Work out the finished part from the listing and answer in its coordinate system (mm). A direction names the side the tool comes from. Round coordinates to 2 decimals unless told otherwise and drop trailing zeros. Order: outer loops, then holes, each group sorted by start corner. A loop starts at its lowest first (then second) coordinate and runs counter-clockwise, first axis right, second up. Notation, with made-up numbers: (32.25, -3.75) - (70.25, -3.75) arc R24 ccw to (70.25, 26.25) - close; hole circle Ø10 at (66.25, 69). An arc over 180 degrees is marked (long way). Answer in a Markdown table with one row per item.
Autodesk Inventor part; units mm, degrees
ref_plane "YZ Plane" through (0, 0, 0) normal (1, 0, 0) x (0, 1, 0)
ref_plane "XZ Plane" through (0, 0, 0) normal (0, 1, 0) x (-1, 0, 0)
ref_plane "XY Plane" through (0, 0, 0) normal (0, 0, 1) x (1, 0, 0)
sketch "草图1" plane through (0, 0, 0) normal (0, 0, 1) x (1, 0, 0)
  circle A0 centre (0, 0) radius 24.5
  dimension "d0" = 49
extrude "拉伸1" add sketch "草图1" along normal blind 20
sketch "草图2" plane through (0, 0, 20) normal (0, 0, 1) x (1, 0, 0)
  circle A0 centre (0, 0) radius 20
  dimension "d3" = 40
extrude "拉伸2" add sketch "草图2" along normal blind 5
chamfer "倒角1" distance 5 distance2 3.5 1 edges at (-20, 0, 25) measured on face at (-2.364, 6.2334, 25)
sketch "草图3" plane through (0, 0, 0) normal (0, 0, -1) x (-1, 0, 0)
  circle A0 centre (0, 0) radius 20
  dimension "d9" = 40
extrude "拉伸3" add sketch "草图3" along normal blind 5
chamfer "倒角2" distance 5 distance2 3.5 1 edges at (20, 0, -5) measured on face at (-7.896, -2.3423, -5)
fillet "圆角1" radius 2 2 edges at (-24.5, 0, 0) (-24.5, 0, 20)
sketch "草图4" plane through (0, 0, -5) normal (0, 0, -1) x (-1, 0, 0)
  circle A0 centre (0, 0) radius 10
  line L0 (11.6, 3) -> (9.5394, 3)
  line L1 (9.5394, 3) -> (9.5394, -3)
  line L2 (9.5394, -3) -> (11.6, -3)
  line L3 (11.6, -3) -> (11.6, 3)
  dimension "d16" = 20
  dimension "d17" = 6
  dimension "d18" = 11.6
extrude "拉伸4" cut sketch "草图4" against normal through all
properties part number "砂轮"
1) Find the intervals of material crossed by probe 1 along Y at (x, z) = (0, 9.5); probe 2 along X at (y, z) = (-6.5, 12.75); probe 3 along Y at (x, z) = (8, 13.75), in increasing order. Write a range as from..to.
Filled in:
| item | result |
|---|---|
| probe 1 | y = -24.5..-10, 10..24.5 |
| probe 2 | x = -23.62..-7.6, 7.6..23.62 |
| probe 3 | y = -23.16..-6, 6..23.16 |
2) Find section B-B, the plane y = 0. Give the vertices of the cut face in (x, z), then the cut area to 3 significant figures.
Filled in:
| item | result |
|---|---|
| outline | (-24.5, 2) arc R2 ccw to (-22.5, 0) - (-20, 0) - (-20, -1.5) - (-15, -5) - (-11.6, -5) - (-11.6, 25) - (-15, 25) - (-20, 21.5) - (-20, 20) - (-22.5, 20) arc R2 ccw to (-24.5, 18) - close; (10, -5) - (15, -5) - (20, -1.5) - (20, 0) - (22.5, 0) arc R2 ccw to (24.5, 2) - (24.5, 18) arc R2 ccw to (22.5, 20) - (20, 20) - (20, 21.5) - (15, 25) - (10, 25) - close |
| area | 694 mm^2 |
3) Which of the six approach directions +Z, -Z, +X, -X, +Y, -Y give full straight-line access (tool end or side, diameter ignored) to faces 4 (the face through (4.336, 19.524, -0.74)), 5 (the face through (-20.1, -1.6, 20)), 6 (the face through (-11, 3, 10))?
Filled in:
| item | result |
|---|---|
| face 4 | -Z |
| face 5 | +Z |
| face 6 | +Z, -Z |
4) Each of these flat-tipped pins is pushed along its axis until it touches: pin 1 (8 mm diameter, centred on y = 18.5, z = 21.5, fed in from -X); pin 2 (8 mm diameter, centred on x = -10, z = -0.5, fed in from -Y); pin 3 (18 mm diameter, centred on x = 0, y = 0, fed in from +Z); pin 4 (2.5 mm diameter, centred on x = -10.5, z = 13.5, fed in from -Y). Where does it stop, or does it pass through?
Filled in:
| item | result |
|---|---|
| pin 1 | stops at x = -18.73 |
| pin 2 | stops at y = -23.55 |
| pin 3 | passes through |
| pin 4 | stops at y = -22.69 |
5) The mould has two halves that part along Y. Classify faces 1 (the face through (-11.6, 0, 10)), 2 (the face through (13.17, -20.66, 9.89)), 3 (the face through (-20.1, -1.6, 0)): released by +Y, released by -Y, zero draft, split by the parting line, or undercut.
Filled in:
| item | result |
|---|---|
| face 1 | undercut |
| face 2 | split by the parting line |
| face 3 | zero draft |
6) Find section A-A, the plane x = 0. Give the vertices of the cut face in (y, z).
Filled in:
| item | result |
|---|---|
| outline | (-24.5, 2) arc R2 ccw to (-22.5, 0) - (-20, 0) - (-20, -1.5) - (-15, -5) - (-10, -5) - (-10, 25) - (-15, 25) - (-20, 21.5) - (-20, 20) - (-22.5, 20) arc R2 ccw to (-24.5, 18) - close; (10, -5) - (15, -5) - (20, -1.5) - (20, 0) - (22.5, 0) arc R2 ccw to (24.5, 2) - (24.5, 18) arc R2 ccw to (22.5, 20) - (20, 20) - (20, 21.5) - (15, 25) - (10, 25) - close |
7) Find section C-C, the plane z = 7.25. Give the vertices of the cut face in (x, y).
Filled in:
| item | result |
|---|---|
| outline | circle Ø49 at (0, 0); hole (-11.6, -3) - (-9.54, -3) arc R10 ccw (long way) to (-9.54, 3) - (-11.6, 3) - close |
